```python
from build123d import *

# Parameters (mm, degrees)
RESSALTO_EXTRUS_O1_DEPTH    = 4
ESBO_O2_W                   = 7
ESBO_O2_H                   = 8
ESBO_O2_W_2                 = 4
ESBO_O2_H_2                 = 16
RESSALTO_EXTRUS_O2_DEPTH    = 25
CORTE_EXTRUS_O1_START       = -35
CORTE_EXTRUS_O1_OUTLINE_R   = 1.75
CORTE_EXTRUS_O1_OUTLINE_R_2 = 1
CORTE_EXTRUS_O1_DEPTH       = 35
RESSALTO_EXTRUS_O3_DEPTH    = 17
RESSALTO_EXTRUS_O4_REACH    = 106.553
ESBO_O7_W                   = 4
ESBO_O7_H                   = 5
ESBO_O8_W                   = 15
ESBO_O8_H                   = 3.5
RESSALTO_EXTRUS_O5_DEPTH    = 2.5
CHANFRO1_SIZE               = 6
CHANFRO2_SIZE               = 3
CHANFRO2_SIZE2              = 6.433520762
CHANFRO3_SIZE               = 1.5
CHANFRO3_SIZE2              = 3.216760381


# Read off the part's stored shape, not the designer's step: Corte-extrusão1
with BuildPart() as part:
    # Esboço1 → Ressalto-extrusão1 (new body)
    with BuildSketch(Plane.XY):
        Polygon((-17.5, 0), (17.5, 0), (17.5, -60), (7.5, -100), (-7.5, -100), (-17.5, -60), align=None)
    extrude(amount=RESSALTO_EXTRUS_O1_DEPTH)

    # Esboço2 → Ressalto-extrusão2 (add)
    with BuildSketch(Plane.XY.offset(4)):
        with Locations((14, -54)):
            Rectangle(ESBO_O2_W, ESBO_O2_H)
        with Locations((14, -4)):
            Rectangle(ESBO_O2_W, ESBO_O2_H)
        with Locations((-15.5, -19)):
            Rectangle(ESBO_O2_W_2, ESBO_O2_H_2)
    extrude(amount=RESSALTO_EXTRUS_O2_DEPTH)

    # Corte-extrusão1 outline → Corte-extrusão1 (cut)
    with BuildSketch(Plane(origin=(17.5, 0, 0), x_dir=(0, 0, -1), z_dir=(1, 0, 0)).offset(CORTE_EXTRUS_O1_START)):
        with Locations((-19, -18.985)):
            Circle(CORTE_EXTRUS_O1_OUTLINE_R)
        with BuildLine():
            ThreePointArc((-19, -25.985), (-26, -18.985), (-19, -11.985))
            Line((-19, -11.985), (-4, -11.985))
            Line((-4, -11.985), (-4, -11))
            Line((-4, -11), (-29, -11))
            Line((-29, -11), (-29, -27))
            Line((-29, -27), (-4, -27))
            Line((-4, -27), (-4, -25.985))
            Line((-4, -25.985), (-19, -25.985))
        make_face()
        with Locations((-24, -4.685)):
            Circle(CORTE_EXTRUS_O1_OUTLINE_R_2)
        with Locations((-14, -4.685)):
            Circle(CORTE_EXTRUS_O1_OUTLINE_R_2)
        with Locations((-14, -53.315)):
            Circle(CORTE_EXTRUS_O1_OUTLINE_R_2)
        with Locations((-24, -53.315)):
            Circle(CORTE_EXTRUS_O1_OUTLINE_R_2)
    extrude(amount=CORTE_EXTRUS_O1_DEPTH, mode=Mode.SUBTRACT)

    # Esboço6 → Ressalto-extrusão3 (add)
    with BuildSketch(Plane.XZ.offset(100)):
        Polygon((-5, 5), (-5, 8.5), (-4.75, 8.5), (-4.75, 11), (-7.5, 11), (-7.5, 4), (7.5, 4), (7.5, 11), (4.75, 11), (4.75, 8.5), (5, 8.5), (5, 5), align=None)
    extrude(amount=-RESSALTO_EXTRUS_O3_DEPTH)

    # Ressalto-extrusão4: up to this face of the body (flat: up to its plane)
    ressalto_extrus_o4_end = Plane(part.part.faces().sort_by_distance((-6.125, -91.5, 11))[0])
    # Esboço7 → Ressalto-extrusão4 (add, up to the picked face)
    with BuildSketch(Plane.XY.offset(4), mode=Mode.PRIVATE) as ressalto_extrus_o4_sk1:
        with Locations((0, -70.5)):
            Rectangle(ESBO_O7_W, ESBO_O7_H)
    ressalto_extrus_o4_tool1 = split(extrude(ressalto_extrus_o4_sk1.sketch, amount=RESSALTO_EXTRUS_O4_REACH, mode=Mode.PRIVATE), bisect_by=ressalto_extrus_o4_end, keep=Keep.BOTH, mode=Mode.PRIVATE)
    # Esboço7 → Ressalto-extrusão4 (add, up to the picked face)
    with BuildSketch(Plane.XY.offset(4), mode=Mode.PRIVATE) as ressalto_extrus_o4_sk2:
        with Locations((5.5, -85.5)):
            Rectangle(ESBO_O7_W, ESBO_O7_H)
    ressalto_extrus_o4_tool2 = split(extrude(ressalto_extrus_o4_sk2.sketch, amount=RESSALTO_EXTRUS_O4_REACH, mode=Mode.PRIVATE), bisect_by=ressalto_extrus_o4_end, keep=Keep.BOTH, mode=Mode.PRIVATE)
    # Esboço7 → Ressalto-extrusão4 (add, up to the picked face)
    with BuildSketch(Plane.XY.offset(4), mode=Mode.PRIVATE) as ressalto_extrus_o4_sk3:
        with Locations((-5.5, -85.5)):
            Rectangle(ESBO_O7_W, ESBO_O7_H)
    ressalto_extrus_o4_tool3 = split(extrude(ressalto_extrus_o4_sk3.sketch, amount=RESSALTO_EXTRUS_O4_REACH, mode=Mode.PRIVATE), bisect_by=ressalto_extrus_o4_end, keep=Keep.BOTH, mode=Mode.PRIVATE)
    add(ressalto_extrus_o4_tool1.solids().sort_by(Axis((0, -70.5, 4), (0, 0, 1)))[0])
    add(ressalto_extrus_o4_tool2.solids().sort_by(Axis((5.5, -85.5, 4), (0, 0, 1)))[0])
    add(ressalto_extrus_o4_tool3.solids().sort_by(Axis((-5.5, -85.5, 4), (0, 0, 1)))[0])

    # Esboço8 → Ressalto-extrusão5 (add)
    with BuildSketch(Plane.XY.offset(11)):
        with Locations((0, -98.25)):
            Rectangle(ESBO_O8_W, ESBO_O8_H)
        with Locations((0, -85.75)):
            Rectangle(ESBO_O8_W, ESBO_O8_H)
    extrude(amount=-RESSALTO_EXTRUS_O5_DEPTH)

    # Chanfro1
    chanfro1_edges = [part.edges().sort_by_distance(p)[0] for p in [
        (0, -68, 4),
        (10.5, -54, 4),
        (10.5, -4, 4),
        (-15.5, -11.985, 4),
        (-15.5, -25.985, 4),
    ]]
    chamfer(chanfro1_edges, length=CHANFRO1_SIZE)

    # Chanfro2
    chanfro2_edges = [part.edges().sort_by_distance(p)[0] for p in [
        (7.5, -91.5, 4),
        (-7.5, -91.5, 4),
    ]]
    chanfro2_side = [part.faces().sort_by_distance(p)[0] for p in [
        (-0.271595018, -42.597184947, 4),
    ]]
    chamfer(chanfro2_edges, length=CHANFRO2_SIZE, length2=CHANFRO2_SIZE2, reference=chanfro2_side[0])

    # Chanfro3
    chanfro3_edges = [part.edges().sort_by_distance(p)[0] for p in [
        (0, -100, 0),
    ]]
    chanfro3_side = [part.faces().sort_by_distance(p)[0] for p in [
        (7.313989248, -100, 10.716760381),
    ]]
    chamfer(chanfro3_edges, length=CHANFRO3_SIZE, length2=CHANFRO3_SIZE2, reference=chanfro3_side[0])


solid = part.part
```
Build history of the part. All positions in model axes, mm. A direction names the side the tool comes from. Coordinates: 2 decimals unless noted, no trailing zeros. Order: outer loops, then holes, each group sorted by start corner. A loop starts at its lowest first (then second) coordinate and runs counter-clockwise, first axis right, second up. Notation, with made-up numbers: (64.5, 82) -> (109.5, 82) arc R17 ccw to (109.5, 99) -> close; hole circle Ø4 at (17, 57.25). An arc over 180 degrees is marked (long way). Answer in a Markdown table with one row per item. Add a question column.
Q1. Mould opens along Y. For faces 1 (the face through (-12.43, -80.28, 2.83)), 2 (the face through (4.75, -92, 10)), 3 (the face through (-13.5, -19, 12)) say: +Y half, -Y half, draft (parallel to the pull), parting line (faces both ways), or undercut.
Q2. Band-saw the part on B-B, the plane z = 14. List the corners of the cut face in (x, y) (3 decimals).
Q3. Which spindle directions (+Z, -Z, +X, -X, +Y, -Y) get a long thin tool onto all of the face, cutting with end or side? Do faces 4 (the face through (-2, -69, 7)), 5 (the face through (-5, -94, 7)), 6 (the face through (14, -50, 16)). Say none if no direction does.
Q4. Band-saw the part on C-C, the plane z = 24. List the corners of the cut face in (x, y) (3 decimals), then the cut area to 3 significant figures.
Q5. Drop flat-ended pins along their axis: pin 1 (8 mm diameter, centred on x = -7, z = 10.5, fed in from +Y); pin 2 (1.5 mm diameter, centred on y = -85, z = 6.5, fed in from -X); pin 3 (1.5 mm diameter, centred on y = -85, z = 6.5, fed in from +X); pin 4 (1.6 mm diameter, centred on y = -53.315, z = 14, fed in from -X). Give the stop position or say it passes through.
Q6. Band-saw the part on D-D, the plane x = 9.5. List the corners of the cut face in (y, z), then the cut area to 3 significant figures.
Q7. Wall check: line 1 along Y through (x, z) = (13, 24) (3 decimals); line 2 along Y through (x, z) = (-14.5, 19) (3 decimals); line 3 along Z through (x, y) = (-3, -7). Give the ranges that are in metal, low to high. Write a range as [from, to].
Q8. Band-saw the part on A-A, the plane x = 0. List the corners of the cut face in (y, z), then the cut area to 3 significant figures.
Answers follow:
| question | item | result |
|---|---|---|
| 1 | face 1 | -Y half |
| 1 | face 2 | undercut |
| 1 | face 3 | draft |
| 2 | outline | (-17.5, -25.985) -> (-13.5, -25.985) -> (-13.5, -11.985) -> (-17.5, -11.985) -> close; (10.5, -58) -> (17.5, -58) -> (17.5, -54.315) -> (10.5, -54.315) -> close; (10.5, -52.315) -> (17.5, -52.315) -> (17.5, -50) -> (10.5, -50) -> close; (10.5, -8) -> (17.5, -8) -> (17.5, -5.685) -> (10.5, -5.685) -> close; (10.5, -3.685) -> (17.5, -3.685) -> (17.5, 0) -> (10.5, 0) -> close |
| 3 | face 4 | +Z, -X, +Y |
| 3 | face 5 | -Y |
| 3 | face 6 | +Z, +X, -X |
| 4 | outline | (-17.5, -23.884) -> (-13.5, -23.884) -> (-13.5, -14.086) -> (-17.5, -14.086) -> close; (10.5, -58) -> (17.5, -58) -> (17.5, -54.315) -> (10.5, -54.315) -> close; (10.5, -52.315) -> (17.5, -52.315) -> (17.5, -50) -> (10.5, -50) -> close; (10.5, -8) -> (17.5, -8) -> (17.5, -5.685) -> (10.5, -5.685) -> close; (10.5, -3.685) -> (17.5, -3.685) -> (17.5, 0) -> (10.5, 0) -> close |
| 4 | area | 123 mm^2 |
| 5 | pin 1 | y = -83 |
| 5 | pin 2 | x = -9.68 |
| 5 | pin 3 | x = 9.68 |
| 5 | pin 4 | through |
| 6 | outline | (-92, 0) -> (0, 0) -> (0, 9) -> (-8, 9) -> (-8, 4) -> (-50, 4) -> (-50, 9) -> (-58, 9) -> (-58, 4) -> (-83, 4) -> (-83, 6.14) -> (-92, 6.14) -> close |
| 6 | area | 467 mm^2 |
| 7 | line 1 | [-58, -54.315], [-52.315, -50], [-8, -5.685], [-3.685, 0] |
| 7 | line 2 | [-25.985, -20.735], [-17.235, -11.985] |
| 7 | line 3 | [0, 4] |
| 8 | outline | (-100, 1.5) -> (-96.78, 0) -> (0, 0) -> (0, 4) -> (-62, 4) -> (-68, 10) -> (-68, 11) -> (-73, 11) -> (-73, 4) -> (-83, 4) -> (-83, 5) -> (-100, 5) -> close; (-100, 8.5) -> (-96.5, 8.5) -> (-96.5, 11) -> (-100, 11) -> close; (-87.5, 8.5) -> (-84, 8.5) -> (-84, 11) -> (-87.5, 11) -> close |
| 8 | area | 485 mm^2 |
